Geometry: final body of the model. Coordinates: model frame, mm. Give positions to 0.01 mm unless a question says otherwise; leave off trailing zeros. Write each loop counter-clockwise with the first axis right and the second up, starting at its lowest first coordinate (ties: lowest second). Pieces come first, ordered by that corner, then holes.
Q1. Cut plane B-B on x = 43.5. Return the cut outline in (y, z) (3 decimals), plus the area to 3 significant figures.
Q2. Cut plane C-C on x = 95.5. Return the cut outline in (y, z), plus the area to 3 significant figures.
Q3. Line query: L1, parallel to Z at x = 66, y = 2.35; L2, parallel to X at y = 4.7, z = -4; L3, parallel to X at y = 1.6, z = -21. Output: solid intervals per line, ascending.
Q4. Cut plane A-A on z = 0. Return the cut outline in (x, y) (3 decimals).
Q5. Pin query (flat end, axial travel): pin 1 (2.5 mm diameter, centred on y = 2.5, z = 10, fed in from +X). Return the tip coordinate at first contact, or that it passes through.
Q6. Cut plane D-D on y = 2.75. Count the separate pieces of the cut face and the enclosed holes in it, plus the area to 3 significant figures.
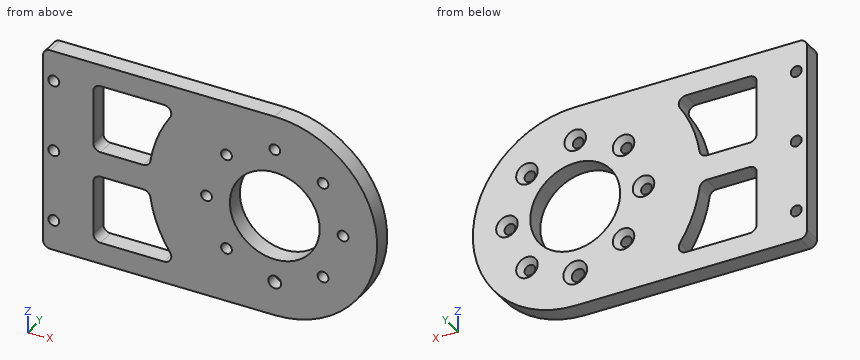
```python
from build123d import *

# Parameters (mm, degrees)
EXTRUDE_1_DEPTH              = 5
SKETCH_2_R                   = 1.275
CUT_EXTRUDE_1_DEPTH          = 6
SKETCH_5_R                   = 10
CUT_EXTRUDE_3_DEPTH          = 6
SKETCH_6_R                   = 1.525
CUT_EXTRUDE_4_DEPTH          = 6
SKETCH_9_R                   = 12.5
CUT_EXTRUDE_7_DEPTH          = 6
HOLE_WIZARD_M3_1_D           = 3.6
HOLE_WIZARD_M3_1_CSINK_D     = 6.6
HOLE_WIZARD_M3_1_CSINK_ANGLE = 90
HOLE_WIZARD_1_D              = 3
HOLE_WIZARD_1_CSINK_D        = 6
HOLE_WIZARD_1_CSINK_ANGLE    = 90
SKETCH_3_R                   = 2.025
CUT_EXTRUDE_8_DEPTH          = 10
SKETCH_14_R                  = 37
EXTRUDE_2_DEPTH              = 5
SKETCH_15_R                  = 42.5
EXTRUDE_3_DEPTH              = 5
SKETCH_16_R                  = 2.025
CUT_EXTRUDE_9_DEPTH          = 5
CUT_EXTRUDE_10_DEPTH         = 5
PATTERN_CIRCULAR_1_COUNT     = 6
SKETCH_19_R                  = 6
CUT_EXTRUDE_11_DEPTH         = 5
FILLET_1_R                   = 2
SKETCH_21_W                  = 189.416251563
SKETCH_21_H                  = 140.293779685
CUT_EXTRUDE_12_DEPTH         = 6
SKETCH_25_R                  = 1.525
CUT_EXTRUDE_13_DEPTH         = 6
FILLET_2_R                   = 2
CUT_EXTRUDE_14_DEPTH         = 6
FILLET_3_R                   = 2


with BuildPart() as part:
    # 草图1 → 凸台-拉伸1 (new body)
    with BuildSketch(Plane(origin=(0, 0, 0), x_dir=(1, 0, 0), z_dir=(0, 1, 0))):
        with BuildLine():
            Line((105, 28.5), (-81.404449572, 28.5))
            ThreePointArc((-81.404449572, 28.5), (-142, 0), (-81.404449572, -28.5))
            Line((-81.404449572, -28.5), (105, -28.5))
            ThreePointArc((105, -28.5), (133.5, 0), (105, 28.5))
        make_face()
    extrude(amount=EXTRUDE_1_DEPTH)

    # 草图2 → 切除-拉伸1 (cut, through all)
    with BuildSketch(Plane.XZ):
        with Locations((118.435028843, 13.435028843)):
            Circle(SKETCH_2_R)
        with Locations((118.435028843, -13.435028843)):
            Circle(SKETCH_2_R)
        with Locations((91.564971157, -13.435028843)):
            Circle(SKETCH_2_R)
        with Locations((91.564971157, 13.435028843)):
            Circle(SKETCH_2_R)
        with Locations((124, 0)):
            Circle(SKETCH_2_R)
        with Locations((105, -19)):
            Circle(SKETCH_2_R)
        with Locations((86, 0)):
            Circle(SKETCH_2_R)
        with Locations((105, 19)):
            Circle(SKETCH_2_R)
    extrude(amount=-CUT_EXTRUDE_1_DEPTH, mode=Mode.SUBTRACT)

    # 草图5 → 切除-拉伸3 (cut, through all)
    with BuildSketch(Plane(origin=(0, 5, 0), x_dir=(1, 0, 0), z_dir=(0, 1, 0))):
        with Locations((-105, 0)):
            Circle(SKETCH_5_R)
    extrude(amount=-CUT_EXTRUDE_3_DEPTH, mode=Mode.SUBTRACT)

    # 草图6 → 切除-拉伸4 (cut, through all)
    with BuildSketch(Plane(origin=(0, 5, 0), x_dir=(1, 0, 0), z_dir=(0, 1, 0))):
        with Locations((-135, 0)):
            Circle(SKETCH_6_R)
        with Locations((-120, 25.980762114)):
            Circle(SKETCH_6_R)
        with Locations((-90, 25.980762114)):
            Circle(SKETCH_6_R)
        with Locations((-75, 0)):
            Circle(SKETCH_6_R)
        with Locations((-90, -25.980762114)):
            Circle(SKETCH_6_R)
        with Locations((-120, -25.980762114)):
            Circle(SKETCH_6_R)
    extrude(amount=-CUT_EXTRUDE_4_DEPTH, mode=Mode.SUBTRACT)

    # 草图9 → 切除-拉伸7 (cut, through all)
    with BuildSketch(Plane.XZ):
        with Locations((105, 0)):
            Circle(SKETCH_9_R)
    extrude(amount=-CUT_EXTRUDE_7_DEPTH, mode=Mode.SUBTRACT)

    # M3 十字槽沉头木螺钉的锥形沉头孔1 (through all)
    with Locations(Plane(origin=(0, 5, 0), x_dir=(1, 0, 0), z_dir=(0, 1, 0))):
        with Locations((105, 19)):
            CounterSinkHole(HOLE_WIZARD_M3_1_D / 2, HOLE_WIZARD_M3_1_CSINK_D / 2, counter_sink_angle=HOLE_WIZARD_M3_1_CSINK_ANGLE)

    # 孔1 (through all)
    with Locations(Plane(origin=(0, 5, 0), x_dir=(1, 0, 0), z_dir=(0, 1, 0))):
        with Locations((91.564971157, 13.435028843), (86, 0), (91.564971157, -13.435028843), (105, -19), (118.435028843, -13.435028843), (124, 0), (118.435028843, 13.435028843)):
            CounterSinkHole(HOLE_WIZARD_1_D / 2, HOLE_WIZARD_1_CSINK_D / 2, counter_sink_angle=HOLE_WIZARD_1_CSINK_ANGLE)

    # 草图3 → 切除-拉伸8 (cut)
    with BuildSketch(Plane(origin=(0, 5, 0), x_dir=(1, 0, 0), z_dir=(0, 1, 0))):
        with Locations((-105, 17.25)):
            Circle(SKETCH_3_R)
        with Locations((-90.061061785, 8.625)):
            Circle(SKETCH_3_R)
        with Locations((-90.061061785, -8.625)):
            Circle(SKETCH_3_R)
        with Locations((-105, -17.25)):
            Circle(SKETCH_3_R)
        with Locations((-119.938938215, -8.625)):
            Circle(SKETCH_3_R)
        with Locations((-119.938938215, 8.625)):
            Circle(SKETCH_3_R)
    extrude(amount=-CUT_EXTRUDE_8_DEPTH, mode=Mode.SUBTRACT)

    # 草图14 → 凸台-拉伸2 (add)
    with BuildSketch(Plane(origin=(0, 5, 0), x_dir=(1, 0, 0), z_dir=(0, 1, 0))):
        with Locations((-105, 0)):
            Circle(SKETCH_14_R)
    extrude(amount=-EXTRUDE_2_DEPTH)

    # 草图15 → 凸台-拉伸3 (add)
    with BuildSketch(Plane(origin=(0, 5, 0), x_dir=(1, 0, 0), z_dir=(0, 1, 0))):
        with Locations((-105, 0)):
            Circle(SKETCH_15_R)
    extrude(amount=-EXTRUDE_3_DEPTH)

    # 草图16 → 切除-拉伸9 (cut)
    with BuildSketch(Plane.XZ):
        with Locations((-105, 26.25)):
            Circle(SKETCH_16_R)
        with Locations((-86.438446994, 18.561553006)):
            Circle(SKETCH_16_R)
        with Locations((-78.75, 0)):
            Circle(SKETCH_16_R)
        with Locations((-86.438446994, -18.561553006)):
            Circle(SKETCH_16_R)
        with Locations((-105, -26.25)):
            Circle(SKETCH_16_R)
        with Locations((-123.561553006, -18.561553006)):
            Circle(SKETCH_16_R)
        with Locations((-131.25, 0)):
            Circle(SKETCH_16_R)
        with Locations((-123.561553006, 18.561553006)):
            Circle(SKETCH_16_R)
    extrude(amount=-CUT_EXTRUDE_9_DEPTH, mode=Mode.SUBTRACT)

    # 草图18 → 切除-拉伸10 (cut)
    with BuildSketch(Plane(origin=(0, 5, 0), x_dir=(1, 0, 0), z_dir=(0, 1, 0))):
        with BuildLine():
            Line((-98.815341562, 17.25), (-101.45814062, 12.173230244))
            ThreePointArc((-101.45814062, 12.173230244), (-105, 13), (-108.54185938, 12.173230244))
            Line((-108.54185938, 12.173230244), (-111.184658438, 17.25))
            ThreePointArc((-111.184658438, 17.25), (-105, 21.75), (-98.815341562, 17.25))
        make_face()
    cut_extrude_10 = extrude(amount=-CUT_EXTRUDE_10_DEPTH, mode=Mode.SUBTRACT)

    # 阵列(圆周)1: 切除-拉伸10 ×6 about axis
    pattern_circular_1_axis = Axis((-105, 0, 0), (0, 1, 0))
    for i in range(1, PATTERN_CIRCULAR_1_COUNT):
        add(cut_extrude_10.rotate(pattern_circular_1_axis, i * 360 / PATTERN_CIRCULAR_1_COUNT), mode=Mode.SUBTRACT)

    # 草图19 → 切除-拉伸11 (cut)
    with BuildSketch(Plane.XZ):
        with Locations((-105, 0)):
            Circle(SKETCH_19_R)
    extrude(amount=-CUT_EXTRUDE_11_DEPTH, mode=Mode.SUBTRACT)

    # 圆角1
    fillet_1_edges = [part.edges().sort_by_distance(p)[0] for p in [
        (-73.472234459, 2.5, 28.5),
        (-73.472234459, 2.5, -28.5),
    ]]
    fillet(fillet_1_edges, radius=FILLET_1_R)

    # 草图21 → 切除-拉伸12 (cut, through all)
    with BuildSketch(Plane.XZ):
        with Locations((-54.208125782, -1.277184269)):
            Rectangle(SKETCH_21_W, SKETCH_21_H)
    extrude(amount=-CUT_EXTRUDE_12_DEPTH, mode=Mode.SUBTRACT)

    # 草图25 → 切除-拉伸13 (cut, through all)
    with BuildSketch(Plane.XZ):
        with Locations((43.5, 0)):
            Circle(SKETCH_25_R)
        with Locations((43.5, 20)):
            Circle(SKETCH_25_R)
        with Locations((43.5, -20)):
            Circle(SKETCH_25_R)
    extrude(amount=-CUT_EXTRUDE_13_DEPTH, mode=Mode.SUBTRACT)

    # 圆角2
    fillet_2_edges = [part.edges().sort_by_distance(p)[0] for p in [
        (40.5, 2.5, -28.5),
        (40.5, 2.5, 28.5),
    ]]
    fillet(fillet_2_edges, radius=FILLET_2_R)

    # 草图28 → 切除-拉伸14 (cut, through all)
    with BuildSketch(Plane.XZ):
        with BuildLine():
            ThreePointArc((70.175439701, 3.5), (72.751903077, 13.603684973), (78.190486763, 22.5))
            Line((78.190486763, 22.5), (54.5, 22.5))
            Line((54.5, 22.5), (54.5, 3.5))
            Line((54.5, 3.5), (70.175439701, 3.5))
        make_face()
        with BuildLine():
            Line((54.5, -3.5), (54.5, -22.5))
            Line((54.5, -22.5), (78.190486763, -22.5))
            ThreePointArc((78.190486763, -22.5), (72.751903077, -13.603684973), (70.175439701, -3.5))
            Line((70.175439701, -3.5), (54.5, -3.5))
        make_face()
    extrude(amount=-CUT_EXTRUDE_14_DEPTH, mode=Mode.SUBTRACT)

    # 圆角3
    fillet_3_edges = [part.edges().sort_by_distance(p)[0] for p in [
        (78.190486763, 2.5, 22.5),
        (70.175439701, 2.5, 3.5),
        (54.5, 2.5, 3.5),
        (54.5, 2.5, 22.5),
        (70.175439701, 2.5, -3.5),
        (78.190486763, 2.5, -22.5),
        (54.5, 2.5, -22.5),
        (54.5, 2.5, -3.5),
    ]]
    fillet(fillet_3_edges, radius=FILLET_3_R)


solid = part.part
```
Data:
1. outline: (0, -28.5) - (5, -28.5) - (5, -21.525) - (0, -21.525) - close; (0, -18.475) - (5, -18.475) - (5, -1.525) - (0, -1.525) - close; (0, 1.525) - (5, 1.525) - (5, 18.475) - (0, 18.475) - close; (0, 21.525) - (5, 21.525) - (5, 28.5) - (0, 28.5) - close
1. area: 239 mm2
2. outline: (0, -28.5) - (5, -28.5) - (5, -8.12) - (0, -8.12) - close; (0, 8.12) - (5, 8.12) - (5, 28.5) - (0, 28.5) - close
2. area: 204 mm2
3. L1: z = -28.5 to -22.5, -3.5 to 3.5, 22.5 to 28.5
3. L2: x = 40.5 to 55.18, 69.73 to 93.16, 116.84 to 133.22
3. L3: x = 40.5 to 42.35, 44.65 to 54.56, 76.13 to 124.27
4. outline: (40.5, 0) - (41.975, 0) - (41.975, 5) - (40.5, 5) - close; (45.025, 0) - (84.5, 0) - (84.5, 3.5) - (83, 5) - (45.025, 5) - close; (87.5, 0) - (92.5, 0) - (92.5, 5) - (89, 5) - (87.5, 3.5) - close; (117.5, 0) - (122.5, 0) - (122.5, 3.5) - (121, 5) - (117.5, 5) - close; (125.5, 0) - (133.5, 0) - (133.5, 5) - (127, 5) - (125.5, 3.5) - close
5. pin 1: stops at x = 132.12
6. separate pieces: 1
6. enclosed holes: 14
6. area: 3,680 mm2
